Work out the finished part from the listing and answer in its coordinate system (mm). A direction names the side the tool comes from. Coordinates: 2 decimals unless noted, no trailing zeros. Order: outer loops, then holes, each group sorted by start corner. A loop starts at its lowest first (then second) coordinate and runs counter-clockwise, first axis right, second up. Notation, with made-up numbers: (66, 40.25) - (99, 40.25) arc R17 cw to (99, 67.25) - close; hole circle Ø2 at (-35, -24.75). An arc over 180 degrees is marked (long way). Answer as a JSON object with one key per item and string values. Group by question number.
1) Section B-B (y = -2.75) is taken. Give the vertices of the cut face in (x, z), plus the area to 3 significant figures.
2) Each of these flat-tipped pins is pushed along its axis until it touches: P1, Ø4, axis at x = 6, z = 10.5, coming from the -Y side; P2, Ø7, axis at x = 7, z = 0, coming from the +Y side; P3, Ø1.1, axis at x = 6, y = -6, coming from the -Z side. Where does it stop, or does it pass through?
3) Find the intervals of material crossed by line 1 along X through (y, z) = (-6.35, 0); line 2 along Z through (x, y) = (7, -1.1); line 3 along Z through (x, y) = (7, -6.25), in increasing order.
4) Section C-C (x = 7) is taken. Give the vertices of the cut face in (y, z).
5) A tool of negligible diameter and unlimited length cuts with its end or side. For faces 4 (the face through (7, -6, 6.2)), 5 (the face through (8.3, -3, -37)), 6 (the face through (5, -5.2, -28)), 7 (the face through (9.2, -5, 2.2)), from which of +Z, -Z, +X, -X, +Y, -Y can it reach the whole face along a straight path? Write none if from no direction.
6) Section D-D (z = -42) is taken. Give the vertices of the cut face in (x, y), plus the area to 3 significant figures.
7) The mould has two halves that part along Z. Classify faces 1 (the face through (7, -5.2, 10)), 2 (the face through (6.971, -2.564, -25.394)), 3 (the face through (7, -3, -49.95)): released by +Z, released by -Z, zero draft, split by the parting line, or undercut.
8) Section A-A (z = 0) is taken. Give the vertices of the cut face in (x, y), plus the area to 3 significant figures.
Autodesk Inventor part; units mm, degrees
ref_plane "YZ Plane" through (0, 0, 0) normal (1, 0, 0) x (0, 1, 0)
ref_plane "XZ Plane" through (0, 0, 0) normal (0, 1, 0) x (-1, 0, 0)
ref_plane "XY Plane" through (0, 0, 0) normal (0, 0, 1) x (1, 0, 0)
sketch "Sketch1" plane through (0, 0, 0) normal (1, 0, 0) x (0, 1, 0)
  line L0 (0, 13.75) -> (-5.2, 13.75)
  line L1 (-5.2, 13.75) -> (-5.2, 6.2)
  line L2 (-5.2, 6.2) -> (-7.4, 6.2)
  line L3 (-7.4, 6.2) -> (-7.4, 2.5)
  line L4 (-7.4, 2.5) -> (-13.4, 2.5) construction
  line L5 (-13.4, 2.5) -> (-13.4, -1.6142) construction
  line L6 (-16.08, 0) -> (2.68, 0) construction
  line L7 (0, -13.75) -> (-5.2, -13.75)
  line L8 (-5.2, -13.75) -> (-5.2, -6.2)
  line L9 (-5.2, -6.2) -> (-7.4, -6.2)
  line L10 (-7.4, -6.2) -> (-7.4, -2.5)
  line L11 (-7.4, -2.5) -> (-13.4, -2.5) construction
  line L12 (-13.4, -2.5) -> (-13.4, -1.6142) construction
  line L13 (0, 13.75) -> (0, -13.75)
  line L14 (-7.4, 2.5) -> (-7.4, -2.5)
  point P0 (0, 0)
  dimension "d1" = 5
  dimension "d2" = 3.7
  dimension "d3" = 6
  dimension "d4" = 2.2
  dimension "d5" = 5.2
  dimension "d52" = 27.5
  dimension "d53" = 7.55
extrude "Extrusion1" add sketch "Sketch1" along normal blind 14
sketch "Sketch2" plane through (0, -5.2, -13.75) normal (0, 0, -1) x (-1, 0, 0)
  line L0 (0, 0) -> (0, 5.2)
  line L1 (0, 5.2) -> (-14, 5.2)
  line L2 (-14, 0) -> (-14, 5.2)
  line L3 (0, 0) -> (-14, 0)
  point P0 (0, 5.2)
sketch "Sketch3" plane through (0, 0, 13.75) normal (0, 1, 0) x (1, 0, 0)
  line L0 (0, 0) -> (14, 0) construction
  line L1 (7, 40.444) -> (7, 60.444) construction
  line L2 (5.7, 40.444) -> (5.7, 60.444)
  line L3 (8.3, 60.444) -> (8.3, 40.444)
  arc A0 (5.7, 40.444) -> (8.3, 40.444) centre (7, 40.444) ccw
  arc A1 (8.3, 60.444) -> (5.7, 60.444) centre (7, 60.444) ccw
  line L4 (0, 69.5) -> (41.7053, 69.5) construction
  circle A2 centre (7, 61.2) radius 2.5 construction
  line L5 (0, 63.7) -> (21.4479, 63.7) construction
  line L6 (-0.0005, 67.5) -> (30.8862, 67.5) construction
  line L7 (0, 27.5) -> (0, 0) construction
  line L8 (7, 0) -> (7, 40.444) construction
  point P0 (7, 50.444)
  dimension "d55" = 2.6
  dimension "d57" = 42
  dimension "d58" = 0.756
  dimension "d59" = 5
  dimension "d60" = 3.8
  dimension "d61" = 2
  dimension "d62" = 20
ref_plane "Work Plane2" through (0, 0, -49.95) normal (0, 0, -1) x (-1, 0, 0)
extrude "Extrusion8" add sketch "Sketch2" along normal up to surface (36.2 mm away)
extrude "Extrusion7" cut sketch "Sketch3" against normal through all
sketch "Sketch5" plane through (0, 0, 13.75) normal (0, 1, 0) x (1, 0, 0)
  point P0 (0, 13.75)
ref_plane "Work Plane1" through (0, -2, 13.75) normal (0, 1, 0) x (1, 0, 0)
sketch "Sketch7" plane through (0, 0, 13.75) normal (0, 1, 0) x (1, 0, 0)
  line L0 (18.6924, 13.75) -> (-14.1545, 13.75) construction
  circle A0 centre (7, 13.75) radius 4.5
  line L1 (14, 0) -> (14, 63.7)
  line L2 (0, 0) -> (14, 0) construction
  line L3 (14, 63.7) -> (-7.462, 63.7) construction
  line L4 (7, 0) -> (7, 13.75) construction
  point P0 (0, 13.75)
  point P1 (3.3, 22.5)
  dimension "d24" = 9
hole "Hole1" at (7, 0, 0) direction (0, -1, 0) diameter 5.5 end through all counterbore diameter 10 counterbore depth 5
properties part number "Sensor_Montage"
Report:
{
 "1": {"outline": "(0, -49.95) - (14, -49.95) - (14, 13.75) - (0, 13.75) - close; hole circle Ø10 at (7, 0); hole (5.7, -46.69) arc R1.3 ccw to (8.3, -46.69) - (8.3, -26.69) arc R1.3 ccw to (5.7, -26.69) - close", "area": "756 mm²"},
 "2": {"P1": "stops at y = -5.2", "P2": "stops at y = -5", "P3": "stops at z = -6.2"},
 "3": {"line 1": "x = 0 to 4.25, 9.75 to 14", "line 2": "z = -49.95 to -47.99, -25.39 to -5, 5 to 13.75", "line 3": "z = -6.2 to -2.75, 2.75 to 6.2"},
 "4": {"outline": "(-7.4, -6.2) - (-5.2, -6.2) - (-5.2, -25.39) - (0, -25.39) - (0, -5) - (-5, -5) - (-5, -2.75) - (-7.4, -2.75) - close; (-7.4, 2.75) - (-5, 2.75) - (-5, 5) - (0, 5) - (0, 13.75) - (-5.2, 13.75) - (-5.2, 6.2) - (-7.4, 6.2) - close; (-5.2, -49.95) - (0, -49.95) - (0, -47.99) - (-5.2, -47.99) - close"},
 "5": {"face 4": "+Z, +X, -X, -Y", "face 5": "+Y, -Y", "face 6": "-Z, +X, -X, -Y", "face 7": "+Y"},
 "6": {"outline": "(0, -5.2) - (5.7, -5.2) - (5.7, 0) - (0, 0) - close; (8.3, -5.2) - (14, -5.2) - (14, 0) - (8.3, 0) - close", "area": "59.3 mm²"},
 "7": {"face 1": "zero draft", "face 2": "undercut", "face 3": "released by -Z"},
 "8": {"outline": "(0, -7.4) - (4.25, -7.4) - (4.25, -5) - (2, -5) - (2, 0) - (0, 0) - close; (9.75, -7.4) - (14, -7.4) - (14, 0) - (12, 0) - (12, -5) - (9.75, -5) - close", "area": "40.4 mm²"}
}
